Model file for the job. Use its own axes, mm. A direction names the side the tool comes from. Coordinates: 2 decimals unless noted, no trailing zeros. Order: outer loops, then holes, each group sorted by start corner. A loop starts at its lowest first (then second) coordinate and runs counter-clockwise, first axis right, second up.
Autodesk Inventor part; units mm, degrees
ref_plane "YZ Plane" through (0, 0, 0) normal (1, 0, 0) x (0, 1, 0)
ref_plane "XZ Plane" through (0, 0, 0) normal (0, 1, 0) x (-1, 0, 0)
ref_plane "XY Plane" through (0, 0, 0) normal (0, 0, 1) x (1, 0, 0)
sketch "Sketch1" plane through (0, 0, 0) normal (0, 1, 0) x (-1, 0, 0)
  line L0 (0, 0) -> (0, -146.336) construction
  line L1 (3, 0) -> (3, -146.336)
  line L2 (-3, -146.336) -> (-3, 0)
  arc A0 (3, 0) -> (-3, 0) centre (0, 0) ccw
  arc A1 (-3, -146.336) -> (3, -146.336) centre (0, -146.336) ccw
  circle A2 centre (0, 0) radius 1.1
  circle A3 centre (0, -146.336) radius 1.1
  circle A4 centre (0, -117.27) radius 1.1
  arc A5 (-3, -117.27) -> (-3, 0) centre (-297.2141, -58.635) ccw
  arc A6 (3, -117.27) -> (3, 0) centre (-291.2141, -58.635) ccw
  point P0 (0, -73.168)
  dimension "d0" = 2.2
  dimension "d1" = 2.2
  dimension "d2" = 6
  dimension "d3" = 146.336
  dimension "d14" = 2.2
  dimension "d15" = 117.27
  dimension "d16" = 300
  dimension "d17" = 300
extrude "Extrusion1" add sketch "Sketch1" along normal blind 4 contours A6 L1 | L1 A1 L2 A5 A0
Q1. Cut at A-A, the plane y = 1.95. List the corners of the cut face in (x, z) (3 decimals).
Established:
outline: (-3, -146.336) arc R3 ccw to (3, -146.336) - (3, -117.27) arc R300 cw to (3, 0) arc R3 ccw to (-3, 0) arc R300 ccw to (-3, -117.27) - close; hole circle Ø2.2 at (0, -146.336); hole circle Ø2.2 at (0, -117.27); hole circle Ø2.2 at (0, 0)
Q2. Which spindle directions (+Z, -Z, +X, -X, +Y, -Y) get a long thin tool onto all of the face, cutting with end or side? Do faces 5 (the face through (3, 2, -132)), 6 (the face through (-3, 2, -132)). Say none if no direction does.
Established:
face 5: +Z, -Z, +X, +Y, -Y
face 6: -Z, -X, +Y, -Y
Q3. Cut at B-B, the plane z = -39. List the corners of the cut face in (x, y).
Established:
outline: (-8.14, 0) - (-2.14, 0) - (-2.14, 4) - (-8.14, 4) - close
Q4. Mould opens along Z. For faces 1 (the face through (-3, 4, -72)), 2 (the face through (-2.785, 1.972, -57.809)), 3 (the face through (-0.066, 1.972, -149.335)), 4 (the face through (0, 2, 3)) say: pulls with the +Z half, pulls with the -Z half, needs draft (parallel to the pull), parting line crosses it, or undercut.
Established:
face 1: needs draft
face 2: undercut
face 3: pulls with the -Z half
face 4: pulls with the +Z half
Q5. Drop flat-ended pins along their axis: P1, Ø1.8, axis at x = 0, z = 0, coming from the -Y side; P2, Ø1.5, axis at y = 3.5, z = -22.5, coming from the +X side. Give the stop position or say it passes through.
Established:
P1: passes through
P2: stops at x = -0.51
Q6. Probe line 1 (X direction, y = 3, z = -117.27); line 2 (X direction, y = 2.2, z = -124); line 3 (X direction, y = 3.7, z = -110.5). List the from-to ranges inside material, lowest first.
Established:
line 1: x = -3 to -1.1, 1.1 to 3
line 2: x = -3 to 3
line 3: x = -4.27 to 1.73
